```python
from build123d import *

# Parameters (mm, degrees)
F2_R     = 7
F3_DEPTH = 15
F4_SIZE  = 1


with BuildPart() as f1:
    # F0 (on Front) → F1 (revolve)
    with BuildSketch(Plane.XZ):
        Polygon((0, 9), (0, 0), (15, 0), (15, 11), (11, 11), (11, 9), align=None)
    revolve(axis=Axis((7.5, 0, 0), (-1, 0, 0)))

    # F2 (on Right) → F3 (cut)
    with BuildSketch(Plane.YZ):
        Circle(F2_R)
    extrude(amount=F3_DEPTH, mode=Mode.SUBTRACT)

    # F4
    f4_edges = [f1.edges().sort_by_distance(p)[0] for p in [
        (0, 0, -9),
    ]]
    chamfer(f4_edges, length=F4_SIZE)


solid = f1.part
```
Geometry: final body of the model. Coordinates: model frame, mm. A direction names the side the tool comes from. Coordinates: 2 decimals unless noted, no trailing zeros. Order: outer loops, then holes, each group sorted by start corner. A loop starts at its lowest first (then second) coordinate and runs counter-clockwise, first axis right, second up. Notation, with made-up numbers: (-7, 0) - (46, 0) arc R16 cw to (46, 29) - close; hole circle Ø2 at (64.5, 73). An arc over 180 degrees is marked (long way). Return JSON: item names as keys, results as strings. Group by question number.
1. Pull-direction query (Y, two-part tool) for faces 3 (the face through (7.395, 6.466, -2.681)), 4 (the face through (0, -6, 4)), 5 (the face through (5.93, 8.923, -1.172)); classes: pulls with the +Y half, pulls with the -Y half, needs draft (parallel to the pull), parting line crosses it, or undercut.
2. Pin query (flat end, axial travel): pin 1 (8 mm diameter, centred on x = 9.5, z = 8.5, fed in from +Y); pin 2 (2 mm diameter, centred on x = 9, y = -3.5, fed in from -Z); pin 3 (8 mm diameter, centred on x = 1.5, z = 4, fed in from -Y); pin 4 (12.5 mm diameter, centred on y = 0, z = 0, fed in from +X). Return the tip coordinate at first contact, or that it passes through.
3. Cut plane C-C (x = 12.5). Output: boundary loops of the cut face in (y, z).
4. Cut plane A-A (z = 0). Output: boundary loops of the cut face in (x, y).
5. Set-up query: faces 1 (the face through (15, 0.2, -7.2)), 2 (the face through (11, -9, 2)). Return all of +Z, -Z, +X, -X, +Y, -Y with unobstructed straight access to the full face (end or side cutting, diameter ignored); none if empty.
6. Cut plane D-D (x = 7.5). Output: boundary loops of the cut face in (y, z), plus the area to 3 significant figures.
7. Material intervals for line 1 along Z through (x, y) = (5.5, 0.25); line 2 along Z through (x, y) = (0.75, -5.75); line 3 along X through (y, z) = (9.25, 0.75), sorted ascending. Write a range as [from, to].
Resolved:
{
 "1": {"face 3": "undercut", "face 4": "needs draft", "face 5": "parting line crosses it"},
 "2": {"pin 1": "stops at y = 9.9", "pin 2": "stops at z = -8.65", "pin 3": "stops at y = -9", "pin 4": "passes through"},
 "3": {"outline": "circle Ø22 at (0, 0); hole circle Ø14 at (0, 0)"},
 "4": {"outline": "(0, -8) - (1, -9) - (11, -9) - (11, -11) - (15, -11) - (15, -7) - (0, -7) - close; (0, 7) - (15, 7) - (15, 11) - (11, 11) - (11, 9) - (1, 9) - (0, 8) - close"},
 "5": {"face 1": "+Z, -Z, +X, +Y, -Y", "face 2": "-X"},
 "6": {"outline": "circle Ø18 at (0, 0); hole circle Ø14 at (0, 0)", "area": "101 mm²"},
 "7": {"line 1": "z = [-9, -7], [7, 9]", "line 2": "z = [-6.6, -3.99], [3.99, 6.6]", "line 3": "x = [11, 15]"}
}
